Can you work these out from the model? Positions are in its coordinate system, mm. A direction names the side the tool comes from. Give positions to 0.01 mm unless a question says otherwise; leave off trailing zeros. Loops run counter-clockwise (first coordinate to the right, second up) from the corner with the lowest first, then second, coordinate; pieces in that order, holes last. Notation, with made-up numbers: M 23.5,26.5 L 80.5,26.5 A33 ccw 80.5,59.5 Z; hole C 8,-10.75 d4. An arc over 180 degrees is marked long. Answer as a JSON object with one key per item and string values.
```python
from build123d import *

# Parameters (mm, degrees)
SALIENTE_EXTRUIR1_DEPTH   = 5
SALIENTE_EXTRUIR1_2_DEPTH = 5
CROQUIS2_R                = 27.5
SALIENTE_EXTRUIR2_DEPTH   = 8
CROQUIS3_R                = 25.5
CROQUIS3_R_2              = 24
SALIENTE_EXTRUIR3_DEPTH   = 3
CROQUIS4_R                = 24
CORTAR_EXTRUIR1_DEPTH     = 3


with BuildPart() as part:
    # Croquis1 → Saliente-Extruir1 (new body)
    with BuildSketch(Plane(origin=(0, 0, 0), x_dir=(1, 0, 0), z_dir=(0, 1, 0))):
        with BuildLine():
            ThreePointArc((-6.024394544, 23.747771903), (-5.19984533, -23.941838036), (15.332388636, 19.109365733))
            ThreePointArc((15.332388636, 19.109365733), (6.749911309, 8.499710515), (-6.481910722, 5.161659186))
            ThreePointArc((-6.481910722, 5.161659186), (-6.882152879, 5.418254788), (-6.886809038, 5.893663462))
            ThreePointArc((-6.886809038, 5.893663462), (-4.77910195, 10.712326415), (-3.398196642, 15.787269012))
            ThreePointArc((-3.398196642, 15.787269012), (-10.284746472, 11.706352258), (-18.035485402, 9.705228534))
            ThreePointArc((-18.035485402, 9.705228534), (-18.552255418, 10.008822773), (-18.406444405, 10.590165925))
            ThreePointArc((-18.406444405, 10.590165925), (-11.764118021, 16.738249367), (-5.966725479, 23.688765141))
            ThreePointArc((-5.966725479, 23.688765141), (-5.995706248, 23.718125601), (-6.024394544, 23.747771903))
        make_face()
        with BuildLine():
            ThreePointArc((-4.563193765, -2.059824722), (-12.054197272, -9.623389101), (-19.617761652, -2.132385594))
            ThreePointArc((-19.617761652, -2.132385594), (-18.516794481, -1.020754013), (-17.4051629, -2.121721183))
            ThreePointArc((-17.4051629, -2.121721183), (-12.064848376, -7.410803529), (-6.775766031, -2.070489005))
            ThreePointArc((-6.775766031, -2.070489005), (-5.67481204, -0.958870731), (-4.563193765, -2.059824722))
        make_face(mode=Mode.SUBTRACT)
        with BuildLine():
            ThreePointArc((7.93388408, -18.140011178), (0.114097404, -20.519185991), (-7.705689271, -18.140011178))
            ThreePointArc((-7.705689271, -18.140011178), (-7.979292605, -16.752516596), (-6.591798022, -16.478913263))
            ThreePointArc((-6.591798022, -16.478913263), (0.114097404, -18.519185991), (6.819992831, -16.478913263))
            ThreePointArc((6.819992831, -16.478913263), (8.207487413, -16.752516596), (7.93388408, -18.140011178))
        make_face(mode=Mode.SUBTRACT)
        with BuildLine():
            ThreePointArc((18.566554033, -1.822088449), (11.169349937, -9.530541219), (3.772145841, -1.822088449))
            ThreePointArc((3.772145841, -1.822088449), (4.944999806, -0.954199424), (5.812888831, -2.127053389))
            ThreePointArc((5.812888831, -2.127053389), (11.092516644, -7.59016676), (16.372144456, -2.127053389))
            ThreePointArc((16.372144456, -2.127053389), (17.316866775, -0.877366131), (18.566554033, -1.822088449))
        make_face(mode=Mode.SUBTRACT)
    extrude(amount=SALIENTE_EXTRUIR1_DEPTH)



with BuildPart() as body_2:
    # Croquis1 → Saliente-Extruir1 2 (new body)
    with BuildSketch(Plane(origin=(0, 0, 0), x_dir=(1, 0, 0), z_dir=(0, 1, 0))):
        with BuildLine():
            ThreePointArc((-3.237616322, 7.170010781), (7.168200526, 11.242778225), (13.650668654, 20.344759652))
            ThreePointArc((13.650668654, 20.344759652), (7.399029371, 23.35603486), (0.553855765, 24.493738869))
            ThreePointArc((0.553855765, 24.493738869), (-1.528467266, 22.741552063), (-4.248394951, 22.650881235))
            ThreePointArc((-4.248394951, 22.650881235), (-7.499015993, 18.503713558), (-11.043045611, 14.604304504))
            ThreePointArc((-11.043045611, 14.604304504), (-11.096230859, 13.969574186), (-10.482918218, 13.797647311))
            ThreePointArc((-10.482918218, 13.797647311), (-5.775579982, 16.492523924), (-1.716909146, 20.090938058))
            ThreePointArc((-1.716909146, 20.090938058), (-1.149234355, 20.211325601), (-0.850096282, 19.714068884))
            ThreePointArc((-0.850096282, 19.714068884), (-1.814955726, 13.671675172), (-3.739754637, 7.863351432))
            ThreePointArc((-3.739754637, 7.863351432), (-3.684337904, 7.37498369), (-3.237616322, 7.170010781))
        make_face()
    extrude(amount=SALIENTE_EXTRUIR1_2_DEPTH)


with BuildPart() as part_1:
    add(part.part)

    add(body_2.part)  # Saliente-Extruir2 merges body 2
    # Croquis2 → Saliente-Extruir2 (add)
    with BuildSketch(Plane(origin=(0, 0, 0), x_dir=(-1, 0, 0), z_dir=(0, -1, 0))):
        Circle(CROQUIS2_R)
    extrude(amount=SALIENTE_EXTRUIR2_DEPTH)

    # Croquis3 → Saliente-Extruir3 (add)
    with BuildSketch(Plane(origin=(0, -8, 0), x_dir=(-1, 0, 0), z_dir=(0, -1, 0))):
        Circle(CROQUIS3_R)
        Circle(CROQUIS3_R_2, mode=Mode.SUBTRACT)
    extrude(amount=SALIENTE_EXTRUIR3_DEPTH)

    # Croquis4 → Cortar-Extruir1 (cut)
    with BuildSketch(Plane(origin=(0, -8, 0), x_dir=(-1, 0, 0), z_dir=(0, -1, 0))):
        Circle(CROQUIS4_R)
    extrude(amount=-CORTAR_EXTRUIR1_DEPTH, mode=Mode.SUBTRACT)


solid = part_1.part
```
1) Suppose I cut it at D-D, the plane y = -1.5. Write out the boundary of the cut face in (x, z), and give its area (3 significant figures).
Answer list:
{"outline": "C 0,0 d55", "area": "2,380 mm^2"}
2) Please list where these lines run through material, in increasing order: line 1 along Z through (x, y) = (0, -7.25); line 2 along Z through (x, y) = (0, -8.7). Write a range as from..to.
Answer list:
{"line 1": "-27.5..-24, 24..27.5", "line 2": "-25.5..-24, 24..25.5"}
3) Will these pins go through, and if not, where does the flat tip stop? pin 1 Ø4 at (x, z) = (12, 0) entering from -Y; pin 2 Ø3.5 at (x, z) = (3, 19.5) entering from +Y; pin 3 Ø4 at (y, z) = (-9.5, -7.5) entering from +X; pin 4 Ø1 at (x, y) = (-6.5, -9) entering from -Z.
Answer list:
{"pin 1": "y = -5", "pin 2": "y = 5", "pin 3": "x = 26.8", "pin 4": "z = -24.78"}
4) Suppose I cut it at C-C, the plane x = 19.5. Write out the boundary of the cut face in (y, z), and give its area (3 significant figures).
Answer list:
{"outline": "M -11,-16.43 L -8,-16.43 L -8,-19.39 L 0,-19.39 L 0,-14.83 L 5,-14.83 L 5,14.83 L 0,14.83 L 0,19.39 L -8,19.39 L -8,16.43 L -11,16.43 L -11,13.99 L -5,13.99 L -5,-13.99 L -11,-13.99 Z", "area": "389 mm^2"}
5) Suppose I cut it at B-B, the plane z = 0. Write out the boundary of the cut face in (x, y), and give its area (3 significant figures).
Answer list:
{"outline": "M -27.5,-8 L -25.5,-8 L -25.5,-11 L -24,-11 L -24,-5 L 24,-5 L 24,-11 L 25.5,-11 L 25.5,-8 L 27.5,-8 L 27.5,0 L 24.5,0 L 24.5,5 L -24.5,5 L -24.5,0 L -27.5,0 Z", "area": "550 mm^2"}
6) If we mould it in two halves opening along X, with no side actions, what happens to faces 1 (the cylindrical face through (5.961, -3.944, 26.846)), 2 (the cylindrical face through (0.01, 2.46, 18.52)), 3 (the flat face through (-15, -11, 19))? For each: +X half, -X half, draft (parallel to the pull), parting line (faces both ways), or undercut.
Answer list:
{"face 1": "parting line", "face 2": "undercut", "face 3": "draft"}
7) Suppose I cut it at A-A, the plane y = 3.25. Give the number of separate pieces and of enclosed holes in the cut face, and give its area (3 significant figures).
Answer list:
{"separate pieces": "2", "enclosed holes": "3", "area": "1,610 mm^2"}
8) For faces 4 (the flat face through (0, -5, 0)), 5 (the cylindrical face through (-1.492, 2.465, -22.756)), 6 (the cylindrical face through (4.92, 2.46, 0.95)), which set-ups out of +Z, -Z, +X, -X, +Y, -Y let a thin tool reach every point of the face, with its end or its side?
Answer list:
{"face 4": "-Y", "face 5": "-Z, +Y", "face 6": "+Y"}
